Design review of the part built by this model. Coordinates are the model's own, in mm. Give positions to 0.01 mm unless a question says otherwise; leave off trailing zeros. Order: outer loops, then holes, each group sorted by start corner. A loop starts at its lowest first (then second) coordinate and runs counter-clockwise, first axis right, second up. Notation, with made-up numbers: M 32,14.5 L 59,14.5 A13 cw 59,28.5 Z; hole C 10.25,7.25 d11. An arc over 180 degrees is marked long. Put each result on its own line as item: value. Start each with the question number.
from build123d import *

# Parameters (mm, degrees)
BOSS_EXTRUDE1_DEPTH = 10.16
FILLET1_R           = 0.5
SKETCH36_R          = 0.15
CUT_EXTRUDE26_DEPTH = 0.1
SKETCH37_R          = 0.75
CUT_EXTRUDE27_DEPTH = 0.5


with BuildPart() as part:
    # Sketch1 → Boss-Extrude1 (new body)
    with BuildSketch(Plane.XY):
        Polygon((-33.789176406, 21.191188847), (-27.689176406, 21.191188847), (-27.439176406, 18.651188847), (-27.689176406, 16.111188847), (-33.789176406, 16.111188847), (-34.039176406, 18.651188847), align=None)
    extrude(amount=BOSS_EXTRUDE1_DEPTH)

    # Fillet1
    fillet1_edges = [part.edges().sort_by_distance(p)[0] for p in [
        (-33.789176406, 21.191188847, 5.08),
        (-27.689176406, 21.191188847, 5.08),
        (-27.689176406, 16.111188847, 5.08),
        (-33.789176406, 16.111188847, 5.08),
    ]]
    fillet(fillet1_edges, radius=FILLET1_R)

    # Sketch36 → Cut-Extrude26 (cut)
    with BuildSketch(Plane(origin=(0, 21.191188847, 0), x_dir=(1, 0, 0), z_dir=(0, 1, 0))):
        with Locations((-32.962004814, -0.994910083)):
            Circle(SKETCH36_R)
    extrude(amount=-CUT_EXTRUDE26_DEPTH, mode=Mode.SUBTRACT)

    # Sketch37 → Cut-Extrude27 (cut)
    with BuildSketch(Plane(origin=(0, 21.191188847, 0), x_dir=(1, 0, 0), z_dir=(0, 1, 0))):
        with Locations((-30.739176406, -10.16)):
            Circle(SKETCH37_R)
    extrude(amount=-CUT_EXTRUDE27_DEPTH, mode=Mode.SUBTRACT)


solid = part.part
1. Insertion check: pin 1 (1 mm diameter, centred on y = 20, z = 7, fed in from +X); pin 2 (2 mm diameter, centred on y = 18.5, z = 8.5, fed in from -X). Each pin has a flat end and moves straight along its axis. Give the tip position at first contact, or say it passes through.
2. Consider section A-A on z = 2.25. Give the boundary of the cut face in (x, y), then the cut area to 3 significant figures.
3. To check wall thickness, follow probe 1 along Y at (x, z) = (-31, 9.5); probe 2 along X at (y, z) = (16.8, 4); probe 3 along Y at (x, z) = (-28, 0.5). State the ranges of each line that lie inside material, in increasing order.
4. Consider section B-B on y = 17.2. Give the boundary of the cut face in (x, z), then the cut area to 3 significant figures.
5. Consider section C-C on x = -27.75. Give the boundary of the cut face in (y, z).
Returned:
1. pin 1: stops at x = -27.52
1. pin 2: stops at x = -34.04
2. outline: M -34.04,18.65 L -33.83,16.56 A0.5 ccw -33.34,16.11 L -28.14,16.11 A0.5 ccw -27.64,16.56 L -27.44,18.65 L -27.64,20.74 A0.5 ccw -28.14,21.19 L -33.34,21.19 A0.5 ccw -33.83,20.74 Z
2. area: 32.1 mm2
3. probe 1: y = 16.11 to 20.69
3. probe 2: x = -33.86 to -27.62
3. probe 3: y = 16.13 to 21.17
4. outline: M -33.9,0 L -27.58,0 L -27.58,10.16 L -33.9,10.16 Z
4. area: 64.2 mm2
5. outline: M 16.3,0 L 21,0 L 21,10.16 L 16.3,10.16 Z
